Read the model definition and answer for the solid it produces. Units are mm, in the model's axes. A direction names the side the tool comes from. Coordinates: 2 decimals unless noted, no trailing zeros. Loops run counter-clockwise (first coordinate to the right, second up) from the corner with the lowest first, then second, coordinate; pieces in that order, holes last.
Autodesk Inventor part; units mm, degrees
ref_plane "YZ Plane" through (0, 0, 0) normal (1, 0, 0) x (0, 1, 0)
ref_plane "XZ Plane" through (0, 0, 0) normal (0, 1, 0) x (-1, 0, 0)
ref_plane "XY Plane" through (0, 0, 0) normal (0, 0, 1) x (1, 0, 0)
sketch "Sketch1" plane through (0, 0, 0) normal (0, 0, 1) x (1, 0, 0)
  line L0 (-33.7638, 59.8408) -> (17.0362, 59.8408)
  line L1 (17.0362, 59.8408) -> (17.0362, -16.3592)
  line L2 (17.0362, -16.3592) -> (-33.7638, -16.3592)
  line L3 (-33.7638, -16.3592) -> (-33.7638, 59.8408)
  dimension "d0" = 50.8
  dimension "d1" = 76.2
extrude "Extrusion1" add sketch "Sketch1" along normal blind 8.89
sketch "Sketch2" plane through (0, 0, 8.89) normal (0, 0, 1) x (1, 0, 0)
  line L0 (17.0362, 59.8408) -> (17.0362, -16.3592)
  line L1 (-33.7638, 59.8408) -> (17.0362, 59.8408)
  line L2 (17.0362, -16.3592) -> (-33.7638, -16.3592)
  line L3 (9.4162, 59.8408) -> (9.4162, -16.3592)
  dimension "d4" = 7.62
extrude "Extrusion2" add sketch "Sketch2" along normal blind 19.05
sketch "Sketch3" plane through (0, 0, 8.89) normal (0, 0, 1) x (1, 0, 0)
  point P0 (9.4162, -16.3592)
  point P1 (-33.7638, -16.3592)
  point P2 (-9.6338, -8.7392)
  point P3 (-25.6982, -1.1192)
  dimension "d7" = 19.05
  dimension "d8" = 7.62
  dimension "d9" = 17.78
  dimension "d10" = 15.24
hole "Hole1" at (-9.6338, -8.7392, 8.89) at (-25.6982, -1.1192, 8.89) direction (0, 0, -1) diameter 2.54 depth 12.7 tip angle 118
sketch "Sketch4" plane through (0, 0, 8.89) normal (0, 0, 1) x (1, 0, 0)
  line L0 (9.4162, -16.3592) -> (9.4162, 59.8408)
  line L1 (-33.7638, 59.8408) -> (9.4162, 59.8408)
  line L2 (-15.9838, 59.8408) -> (-15.9838, 9.0408)
  line L3 (-15.9838, 9.0408) -> (-3.2838, 9.0408)
  line L4 (-3.2838, 9.0408) -> (-3.2838, 59.8408)
  dimension "d18" = 12.7
  dimension "d19" = 12.7
  dimension "d22" = 50.8
extrude "Extrusion3" add sketch "Sketch4" along normal up to surface (19.05 mm away)
properties part number "base"
Item 1: A cutting plane is placed at C-C on x = -5. Determine the outline of the cut face in (y, z).
Numbers:
outline: (-16.36, 0) - (59.84, 0) - (59.84, 27.94) - (9.04, 27.94) - (9.04, 8.89) - (-16.36, 8.89) - close
Item 2: Find the intervals of material crossed by line 1 along X through (y, z) = (48, 18.75); line 2 along Z through (x, y) = (-7, 9); line 3 along Y through (x, z) = (-6.5, 9.75), in increasing order.
Numbers:
line 1: x = -15.98 to -3.28, 9.42 to 17.04
line 2: z = 0 to 8.89
line 3: y = 9.04 to 59.84
Item 3: A cutting plane is placed at D-D on x = -30. Determine the outline of the cut face in (y, z).
Numbers:
outline: (-16.36, 0) - (59.84, 0) - (59.84, 8.89) - (-16.36, 8.89) - close
Item 4: Determine the mould class of faces 6 (the face through (-24.46, -0.84, 4.38)), 7 (the face through (-17, 22, 8.89)), 8 (the face through (-2, -16.359, 8)), 9 (the face through (-8.51, -9.33, 4.38)) for opening direction Y: released by +Y, released by -Y, zero draft, split by the parting line, or undercut.
Numbers:
face 6: undercut
face 7: zero draft
face 8: released by -Y
face 9: undercut
Item 5: Given pin 1 (5 mm diameter, centred on y = 37.5, z = 12.5, fed in from -X); pin 2 (13 mm diameter, centred on x = -23, y = 4, fed in from +Z); pin 3 (2 mm diameter, centred on x = -25.7, y = -1.12, fed in from -Z); pin 4 (6.5 mm diameter, centred on x = -8, z = 17.5, fed in from -Y), each flat-ended and moving along its own axis, determine where each tip first touches the part or whether it passes through.
Numbers:
pin 1: stops at x = -15.98
pin 2: stops at z = 8.89
pin 3: passes through
pin 4: stops at y = 9.04
Item 6: Which of the six approach directions +Z, -Z, +X, -X, +Y, -Y give full straight-line access (tool end or side, diameter ignored) to faces 1 (the face through (9.416, 22, 18)), 2 (the face through (-9, 22, 0)), 3 (the face through (17.036, 22, 14)), 4 (the face through (-15.984, 35, 18)), 5 (the face through (-10, 9.041, 18))?
Numbers:
face 1: +Z, +Y, -Y
face 2: -Z, +X, -X, +Y, -Y
face 3: +Z, -Z, +X, +Y, -Y
face 4: +Z, -X, +Y, -Y
face 5: +Z, -X, -Y
Item 7: A cutting plane is placed at A-A on z = 10.75. Determine the outline of the cut face in (x, y).
Numbers:
outline: (-15.98, 9.04) - (-3.28, 9.04) - (-3.28, 59.84) - (-15.98, 59.84) - close; (9.42, -16.36) - (17.04, -16.36) - (17.04, 59.84) - (9.42, 59.84) - close
Item 8: A cutting plane is placed at B-B on y = 19.5. Determine the outline of the cut face in (x, z).
Numbers:
outline: (-33.76, 0) - (17.04, 0) - (17.04, 27.94) - (9.42, 27.94) - (9.42, 8.89) - (-3.28, 8.89) - (-3.28, 27.94) - (-15.98, 27.94) - (-15.98, 8.89) - (-33.76, 8.89) - close
